```python
from build123d import *

# Parameters (mm, degrees)
F0_R     = 2.38125
F0_R_2   = 2.032
F1_DEPTH = 3.175


with BuildPart() as f1:
    # F0 (on Right) → F1 (new body)
    with BuildSketch(Plane.YZ):
        with BuildLine():
            ThreePointArc((-4.7625, 152.4), (0, 147.6375), (4.7625, 152.4))
            ThreePointArc((4.7625, 152.4), (0, 157.1625), (-4.7625, 152.4))
        make_face()
        with Locations((0, 152.4)):
            Circle(F0_R, mode=Mode.SUBTRACT)
        with BuildLine():
            Line((4.7625, 0), (4.7625, 152.4))
            ThreePointArc((4.7625, 152.4), (0, 147.6375), (-4.7625, 152.4))
            Line((-4.7625, 152.4), (-4.7625, 0))
            ThreePointArc((-4.7625, 0), (0, -4.7625), (4.7625, 0))
        make_face()
        Circle(F0_R_2, mode=Mode.SUBTRACT)
        with Locations((0, 12.7)):
            Circle(F0_R_2, mode=Mode.SUBTRACT)
    extrude(amount=F1_DEPTH)


solid = f1.part
```
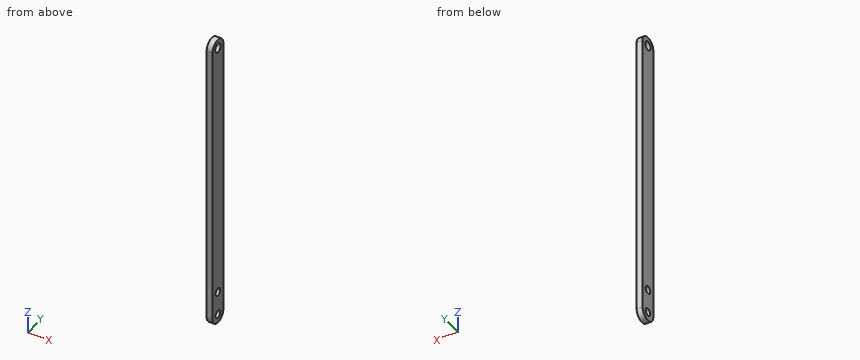
Can you work these out from the model? Positions are in its coordinate system, mm. Coordinates: 2 decimals unless noted, no trailing zeros. Write each loop counter-clockwise with the first axis right and the second up, starting at its lowest first coordinate (ties: lowest second). Pieces come first, ordered by that corner, then holes. Notation, with made-up numbers: (5.25, 13) - (15.25, 13) arc R29 ccw to (15.25, 41) - close; hole circle Ø8 at (-18.5, 44). An arc over 180 degrees is marked (long way). Return JSON: item names as keys, results as strings.
Q1. Please list where these lines run through material, in increasing order: L1, parallel to Z at x = 0.9, y = 0; L2, parallel to Y at x = 1.15, z = 152.4; L3, parallel to Z at x = 2.8, y = -1.5. Write a range as from..to.
Computed values:
{"L1": "z = -4.76..-2.03, 2.03..10.67, 14.73..150.02, 154.78..157.16", "L2": "y = -4.76..-2.38, 2.38..4.76", "L3": "z = -4.52..-1.37, 1.37..11.33, 14.07..150.55, 154.25..156.92"}
Q2. If we section it at B-B (x = 1.25): Please give me the cut outline in (y, z) (1 decimal), then the cut area to 3 significant figures.
Computed values:
{"outline": "(-4.8, 0) arc R4.8 ccw to (4.8, 0) - (4.8, 152.4) arc R4.8 ccw to (-4.8, 152.4) - close; hole circle Ø4.8 at (0, 152.4); hole circle Ø4.1 at (0, 0); hole circle Ø4.1 at (0, 12.7)", "area": "1,480 mm2"}
Q3. If we section it at C-C (z = 12.7): Please give me the cut outline in (x, y) (1 decimal).
Computed values:
{"outline": "(0, -4.8) - (3.2, -4.8) - (3.2, -2) - (0, -2) - close; (0, 2) - (3.2, 2) - (3.2, 4.8) - (0, 4.8) - close"}
Q4. I'm going to push flat-ended pins straight in: pin 1 Ø3.5 at (y, z) = (0, 12.7) entering from +X; pin 2 Ø1 at (x, y) = (2, -1) entering from +Z. Where does each tip first touch, or does it pass through?
Computed values:
{"pin 1": "passes through", "pin 2": "stops at z = 157.14"}
Q5. If we section it at A-A (y = 0): Please give me the cut outline in (x, z) (1 decimal).
Computed values:
{"outline": "(0, -4.8) - (3.2, -4.8) - (3.2, -2) - (0, -2) - close; (0, 2) - (3.2, 2) - (3.2, 10.7) - (0, 10.7) - close; (0, 14.7) - (3.2, 14.7) - (3.2, 150) - (0, 150) - close; (0, 154.8) - (3.2, 154.8) - (3.2, 157.2) - (0, 157.2) - close"}
